from build123d import *

# Parameters (mm, degrees)
F1_DEPTH    = 7.5
F2_SIZE     = 1
F3_T1_DEPTH = 21.6421356237
F4_R        = 1.6
F5_DEPTH    = 5.001
F6_R        = 1.6
F7_DEPTH    = 5.001
F8_R        = 1.6
F9_DEPTH    = 5.001
F10_R       = 2.85
F10_R_2     = 1.6
F11_DEPTH   = 3


# Not quite as in the source:
# - a fillet or chamfer that OpenCascade refuses, or shapes differently, is made with other operations: its cross-section is extruded or revolved along the edge and cut away or added


with BuildPart() as f1:
    # F0 (on Front) → F1 (new body)
    with BuildSketch(Plane.XZ):
        Polygon((0, 10), (0, 0), (35.8, 0), (35.8, 10), (32.8, 10), (32.8, 5), (26.4, 5), (26.4, 10), (21.1, 10), (21.1, 5), (14.7, 5), (14.7, 10), (9.4, 10), (9.4, 5), (3, 5), (3, 10), align=None)
    extrude(amount=F1_DEPTH)

    # F2
    f2_edges = [f1.edges().sort_by_distance(p)[0] for p in [
        (3, -3.75, 10),
        (9.4, -3.75, 10),
        (14.7, -3.75, 10),
        (21.1, -3.75, 10),
        (26.4, -3.75, 10),
        (32.8, -3.75, 10),
    ]]
    chamfer(f2_edges, length=F2_SIZE)

    # F3: fillet of radius 3 on 2 edges, made by hand

    # F3_s2 → F3_t1 (cut)
    with BuildSketch(Plane.XZ.offset(-7.0710678119)):
        with BuildLine():
            ThreePointArc((0, 7.1715728753), (0.5505102572, 8.9036236828), (2, 10))
            Line((2, 10), (0, 10))
            Line((0, 10), (0, 7.1715728753))
        make_face()
        with BuildLine():
            ThreePointArc((33.8, 10), (35.2494897428, 8.9036236828), (35.8, 7.1715728753))
            Line((35.8, 7.1715728753), (35.8, 10))
            Line((35.8, 10), (33.8, 10))
        make_face()
    extrude(amount=F3_T1_DEPTH, mode=Mode.SUBTRACT)

    # F4 (on face) → F5 (cut, through all)
    with BuildSketch(Plane.XY.offset(5)):
        with Locations((6.2, -3.75)):
            Circle(F4_R)
    extrude(amount=-F5_DEPTH, mode=Mode.SUBTRACT)

    # F6 (on face) → F7 (cut, through all)
    with BuildSketch(Plane.XY.offset(5)):
        with Locations((17.9, -3.75)):
            Circle(F6_R)
    extrude(amount=-F7_DEPTH, mode=Mode.SUBTRACT)

    # F8 (on face) → F9 (cut, through all)
    with BuildSketch(Plane.XY.offset(5)):
        with Locations((29.6, -3.75)):
            Circle(F8_R)
    extrude(amount=-F9_DEPTH, mode=Mode.SUBTRACT)

    # F10 (on face) → F11 (cut)
    with BuildSketch(Plane(origin=(0, 0, 0), x_dir=(1, 0, 0), z_dir=(0, 0, -1))):
        with Locations((6.2, 3.75)):
            Circle(F10_R)
        with Locations((6.2, 3.75)):
            Circle(F10_R_2, mode=Mode.SUBTRACT)
        with Locations((17.9, 3.75)):
            Circle(F10_R)
        with Locations((17.9, 3.75)):
            Circle(F10_R_2, mode=Mode.SUBTRACT)
        with Locations((29.6, 3.75)):
            Circle(F10_R)
        with Locations((29.6, 3.75)):
            Circle(F10_R_2, mode=Mode.SUBTRACT)
    extrude(amount=-F11_DEPTH, mode=Mode.SUBTRACT)


solid = f1.part
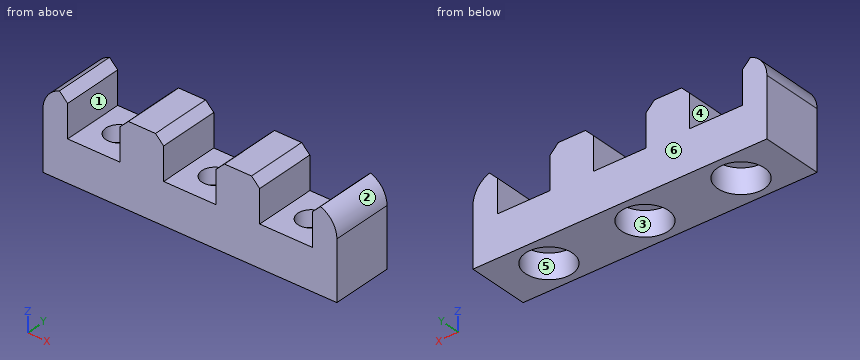
Geometry: final body of the model. Coordinates: model frame, mm. Face numbers are marked on the shaded views. A direction names the side the tool comes from. Coordinates: 2 decimals unless noted, no trailing zeros. Write each loop counter-clockwise with the first axis right and the second up, starting at its lowest first coordinate (ties: lowest second). Pieces come first, ordered by that corner, then holes. Notation, with made-up numbers: (-32, -14.5) - (-4, -14.5) arc R21 ccw to (-4, -10.5) - close; hole circle Ø7 at (-13.5, 34.5). An arc over 180 degrees is marked (long way). Return JSON: item names as keys, results as strings.
Item 1: Pin query (flat end, axial travel): pin 1 Ø3 at (x, y) = (6.2, -3.75) entering from -Z; pin 2 Ø3.5 at (x, y) = (29.6, -3.75) entering from -Z; pin 3 Ø1.9 at (x, y) = (30, -5) entering from +Z. Return the tip coordinate at first contact, or that it passes through.
Completed:
{"pin 1": "passes through", "pin 2": "stops at z = 3", "pin 3": "stops at z = 5"}
Item 2: Line query: L1, parallel to X at y = -3.75, z = 4.4; L2, parallel to X at y = -3.75, z = 2.1; L3, parallel to Y at x = 17.9, z = 4.4. Output: solid intervals per line, ascending.
Completed:
{"L1": "x = 0 to 4.6, 7.8 to 16.3, 19.5 to 28, 31.2 to 35.8", "L2": "x = 0 to 3.35, 9.05 to 15.05, 20.75 to 26.75, 32.45 to 35.8", "L3": "y = -7.5 to -5.35, -2.15 to 0"}
Item 3: Section query D-D (z = 7.5). Output: boundary loops of the cut face in (x, y).
Completed:
{"outline": "(0.02, -7.5) - (3, -7.5) - (3, 0) - (0.02, 0) - close; (9.4, -7.5) - (14.7, -7.5) - (14.7, 0) - (9.4, 0) - close; (21.1, -7.5) - (26.4, -7.5) - (26.4, 0) - (21.1, 0) - close; (32.8, -7.5) - (35.78, -7.5) - (35.78, 0) - (32.8, 0) - close"}
Item 4: Section query C-C (z = 2.25). Output: boundary loops of the cut face in (x, y).
Completed:
{"outline": "(0, -7.5) - (35.8, -7.5) - (35.8, 0) - (0, 0) - close; hole circle Ø5.7 at (6.2, -3.75); hole circle Ø5.7 at (17.9, -3.75); hole circle Ø5.7 at (29.6, -3.75)"}
Item 5: Section query A-A (z = 4.5). Output: boundary loops of the cut face in (x, y).
Completed:
{"outline": "(0, -7.5) - (35.8, -7.5) - (35.8, 0) - (0, 0) - close; hole circle Ø3.2 at (6.2, -3.75); hole circle Ø3.2 at (17.9, -3.75); hole circle Ø3.2 at (29.6, -3.75)"}
Item 6: Section query B-B (x = 29.6). Output: boundary loops of the cut face in (y, z).
Completed:
{"outline": "(-7.5, 0) - (-6.6, 0) - (-6.6, 3) - (-5.35, 3) - (-5.35, 5) - (-7.5, 5) - close; (-2.15, 3) - (-0.9, 3) - (-0.9, 0) - (0, 0) - (0, 5) - (-2.15, 5) - close"}
Item 7: Pull-direction query (Y, two-part tool) for the marked faces 4, 5 and 6; classes: +Y half, -Y half, draft (parallel to the pull), parting line (faces both ways), or undercut.
Completed:
{"face 4": "draft", "face 5": "undercut", "face 6": "+Y half"}
Item 8: Reachability of the marked faces 1, 2 and 3 from +Z, -Z, +X, -X, +Y, -Y: full face, straight path, thin tool, end or side. Return the list, or none.
Completed:
{"face 1": "+Z, +Y, -Y", "face 2": "+Z, +X, +Y, -Y", "face 3": "-Z"}
